Verification items for the finished model (mm, model axes). A direction names the side the tool comes from. Round coordinates to 2 decimals unless told otherwise and drop trailing zeros. Loops run counter-clockwise (first coordinate to the right, second up) from the corner with the lowest first, then second, coordinate; pieces in that order, holes last. Notation, with made-up numbers: (31, 58) -> (36, 58) arc R30 ccw to (36, 85) -> close; hole circle Ø10 at (28.5, -26.5). An arc over 180 degrees is marked (long way). Write item = value, one per line.
```python
from build123d import *


# Not quite as in the source:
# - a feature names something its author has since deleted; it is built from what else it names


with BuildPart() as f1:
    # F0 (on Front) → F1 (revolve)
    with BuildSketch(Plane.XZ):
        with BuildLine():
            Line((0, 7.540625), (0, 12.2555))
            Line((0, 12.2555), (-6.0455628512, 10.6355963162))
            ThreePointArc((-6.0455628512, 10.6355963162), (-7.3184226416, 9.7850985952), (-7.8105, 8.3354854424))
            Line((-7.8105, 8.3354854424), (-7.8105, 6.49986))
            Line((-7.8105, 6.49986), (-4.7625, 6.49986))
            Line((-4.7625, 6.49986), (-4.7625, 7.540625))
            Line((-4.7625, 7.540625), (0, 7.540625))
        make_face()
    revolve(axis=Axis((5.2561350167, 0, 0), (1, 0, 0)))


solid = f1.part
```
(1) Sectioned sample at C-C, the plane x = -1.25. Record the cut outline in (y, z).
Filled sheet:
outline = circle Ø23.84 at (0, 0); hole circle Ø15.08 at (0, 0)
(2) Go/stop test with flat-tipped pins: pin 1 Ø10 at (y, z) = (8, -6.5) entering from -X; pin 2 Ø1.5 at (x, y) = (-1.5, -3) entering from +Z; pin 3 Ø12 at (y, z) = (-0.5, 0.5) entering from +X. Record where each tip stops, or that it passes through.
Filled sheet:
pin_1 = -7.81
pin_2 = 11.74
pin_3 = -4.76
(3) Sectioned sample at D-D, the plane x = -3. Record the cut outline in (y, z).
Filled sheet:
outline = circle Ø22.9 at (0, 0); hole circle Ø15.08 at (0, 0)
(4) Sectioned sample at A-A, the plane y = 0. Record the cut outline in (x, z).
Filled sheet:
outline = (-7.81, -8.34) arc R2.38 ccw to (-6.05, -10.64) -> (0, -12.26) -> (0, -7.54) -> (-4.76, -7.54) -> (-4.76, -6.5) -> (-7.81, -6.5) -> close; (-7.81, 6.5) -> (-4.76, 6.5) -> (-4.76, 7.54) -> (0, 7.54) -> (0, 12.26) -> (-6.05, 10.64) arc R2.38 ccw to (-7.81, 8.34) -> close
(5) Material ranges on probe 1 along Y at (x, z) = (-6, 1.75); probe 2 along Z at (x, y) = (-5.5, -5.25); probe 3 along Z at (x, y) = (-1, -5.5), recorded low to high. Write a range as from..to.
Filled sheet:
probe_1 = -10.5..-6.26, 6.26..10.5
probe_2 = -9.42..-3.83, 3.83..9.42
probe_3 = -10.65..-5.16, 5.16..10.65
(6) Set-up check for faces 1 (the face through (-4.762, -6, -3)), 2 (the face through (0, 5, 6)): record each of +Z, -Z, +X, -X, +Y, -Y from which the full face is reachable in a straight line by a thin tool's end or side.
Filled sheet:
face_1 = +X
face_2 = +Z, -Z, +X, +Y, -Y
(7) Draft check along Y on faces 3 (the face through (-5.75, 10.46, -2.32)), 4 (the face through (-2.348, -0.332, -7.533)), 5 (the face through (-7.811, 6, -3)). Enter one of: released by +Y, released by -Y, zero draft, split by the parting line, or undercut.
Filled sheet:
face_3 = split by the parting line
face_4 = undercut
face_5 = zero draft
